from build123d import *

# Parameters (mm, degrees)
SKETCH1_W           = 13.26865531
SKETCH1_H           = 13.268655309
BOSS_EXTRUDE1_DEPTH = 7.62
SKETCH5_R           = 1.27
CUT_EXTRUDE3_DEPTH  = 8.62
CUT_EXTRUDE5_REACH  = 9.62
SKETCH9_W           = 32
SKETCH9_H           = 8.5
SKETCH10_R          = 1.625
CUT_EXTRUDE6_DEPTH  = 8.62
SKETCH13_W          = 21.59
SKETCH13_H          = 6.35
SKETCH13_W_2        = 13.26865531
BOSS_EXTRUDE2_DEPTH = 19.05
SKETCH14_R          = 2.286
CUT_EXTRUDE7_DEPTH  = 201.924200001
SKETCH15_R          = 2.286
CUT_EXTRUDE8_DEPTH  = 123.971427656
SKETCH8_R           = 1.6250031
CUT_EXTRUDE9_DEPTH  = 27.67
SKETCH19_R          = 2.286
CUT_EXTRUDE13_DEPTH = 201.924200001
CUT_EXTRUDE14_REACH = 28.67
SKETCH20_R          = 1.625
SKETCH22_W          = 11.684
SKETCH22_H          = 11.684
SKETCH22_W_2        = 45.3
SKETCH22_H_2        = 36.3
SKETCH22_W_3        = 83.82
SKETCH22_H_3        = 63.500000001
SKETCH22_W_4        = 41.91
SKETCH22_W_5        = 15.24
SKETCH22_H_4        = 100.5942
CUT_EXTRUDE15_DEPTH = 27.67
SKETCH24_R          = 1.625
CUT_EXTRUDE16_DEPTH = 27.67
FILLET2_R           = 6.35
FILLET4_R           = 6.35
FILLET5_R           = 6.35


with BuildPart() as part:
    # Sketch1 → Boss-Extrude1 (new body)
    with BuildSketch(Plane(origin=(0, 0, 0), x_dir=(-1, 0, 0), z_dir=(0, 0, 1))):
        Polygon((0, -67.741156164), (0, -193.735356164), (-21.59, -193.735356164), (-21.59, -215.325356165), (0, -215.325356165), (0, -240.725356165), (-153.67, -240.725356165), (-153.67, -165.028256165), (-195.58, -165.028256165), (-195.58, -89.331156165), (-217.17, -89.331156165), (-217.17, -67.741156164), (-195.58, -67.741156164), (-195.58, -46.151156164), (-217.17, -46.151156164), (-217.17, -20.751156164), (0, -20.751156164), (0, -46.151156164), (-21.59, -46.151156164), (-21.59, -67.741156164), align=None)
        with Locations((-114.925672351, -130.738256165)):
            Rectangle(SKETCH1_W, SKETCH1_H, mode=Mode.SUBTRACT)
    extrude(amount=BOSS_EXTRUDE1_DEPTH)

    # Sketch5 → Cut-Extrude3 (cut, through all)
    with BuildSketch(Plane.XY.offset(7.62)):
        with Locations((44.45, 234.375356165)):
            Circle(SKETCH5_R)
        with Locations((140.97, 234.375356165)):
            Circle(SKETCH5_R)
        with Locations((44.45, 158.175356164)):
            Circle(SKETCH5_R)
        with Locations((140.97, 158.175356164)):
            Circle(SKETCH5_R)
    extrude(amount=-CUT_EXTRUDE3_DEPTH, mode=Mode.SUBTRACT)

    # Sketch9 → Cut-Extrude5 (cut, up to next)
    with BuildSketch(Plane(origin=(0, 0, 0), x_dir=(-1, 0, 0), z_dir=(0, 0, -1)), mode=Mode.PRIVATE) as cut_extrude5_sk1:
        with Locations((-43.94, 33.467738164)):
            Rectangle(SKETCH9_W, SKETCH9_H)
    cut_extrude5_tool1 = extrude(cut_extrude5_sk1.sketch, amount=-CUT_EXTRUDE5_REACH, mode=Mode.PRIVATE) & part.part
    add(cut_extrude5_tool1.solids().sort_by_distance((43.94, 33.467738, 0))[0], mode=Mode.SUBTRACT)

    # Sketch10 → Cut-Extrude6 (cut, through all)
    with BuildSketch(Plane.XY.offset(7.62)):
        with Locations((179.07, 142.930256164)):
            Circle(SKETCH10_R)
        with Locations((179.07, 118.546256164)):
            Circle(SKETCH10_R)
        with Locations((154.686, 118.546256164)):
            Circle(SKETCH10_R)
        with Locations((154.686, 142.930256164)):
            Circle(SKETCH10_R)
    extrude(amount=-CUT_EXTRUDE6_DEPTH, mode=Mode.SUBTRACT)

    # Sketch13 → Boss-Extrude2 (add)
    with BuildSketch(Plane.XY.offset(7.62)):
        with Locations((10.795, 218.500356165)):
            Rectangle(SKETCH13_W, SKETCH13_H)
        with Locations((10.795, 190.560356164)):
            Rectangle(SKETCH13_W, SKETCH13_H)
        with Locations((10.795, 42.976156164)):
            Rectangle(SKETCH13_W, SKETCH13_H)
        with Locations((10.795, 70.916156164)):
            Rectangle(SKETCH13_W, SKETCH13_H)
        with Locations((114.925672351, 140.547583819)):
            Rectangle(SKETCH13_W_2, SKETCH13_H)
        with Locations((114.925672351, 120.92892851)):
            Rectangle(SKETCH13_W_2, SKETCH13_H)
        with Locations((206.375, 42.976156164)):
            Rectangle(SKETCH13_W, SKETCH13_H)
        with Locations((206.375, 70.916156164)):
            Rectangle(SKETCH13_W, SKETCH13_H)
    extrude(amount=BOSS_EXTRUDE2_DEPTH)

    # Sketch14 → Cut-Extrude7 (cut, through all)
    with BuildSketch(Plane.XZ.offset(-39.801156164)):
        with Locations((10.795, 17.145)):
            Circle(SKETCH14_R)
    extrude(amount=-CUT_EXTRUDE7_DEPTH, mode=Mode.SUBTRACT)

    # Sketch15 → Cut-Extrude8 (cut, through all)
    with BuildSketch(Plane.XZ.offset(-117.75392851)):
        with Locations((114.925672351, 17.145)):
            Circle(SKETCH15_R)
    extrude(amount=-CUT_EXTRUDE8_DEPTH, mode=Mode.SUBTRACT)

    # Sketch8 → Cut-Extrude9 (cut, through all)
    with BuildSketch(Plane(origin=(0, 0, 0), x_dir=(-1, 0, 0), z_dir=(0, 0, -1))):
        with Locations((-88.9, 52.501156164)):
            Circle(SKETCH8_R)
        with Locations((-146.9, 52.501156164)):
            Circle(SKETCH8_R)
        with Locations((-88.9, 101.501156164)):
            Circle(SKETCH8_R)
        with Locations((-146.9, 101.501156164)):
            Circle(SKETCH8_R)
    extrude(amount=-CUT_EXTRUDE9_DEPTH, mode=Mode.SUBTRACT)

    # Sketch19 → Cut-Extrude13 (cut, through all)
    with BuildSketch(Plane.XZ.offset(-39.801156164)):
        with Locations((206.375, 17.145)):
            Circle(SKETCH19_R)
    extrude(amount=-CUT_EXTRUDE13_DEPTH, mode=Mode.SUBTRACT)

    # Sketch20 → Cut-Extrude14 (cut, up to next)
    with BuildSketch(Plane(origin=(0, 0, 0), x_dir=(-1, 0, 0), z_dir=(0, 0, -1)), mode=Mode.PRIVATE) as cut_extrude14_sk1:
        with Locations((-81.741344696, 139.338256164)):
            Circle(SKETCH20_R)
    cut_extrude14_tool1 = extrude(cut_extrude14_sk1.sketch, amount=-CUT_EXTRUDE14_REACH, mode=Mode.PRIVATE) & part.part
    add(cut_extrude14_tool1.solids().sort_by_distance((81.741345, 139.338256, 0))[0], mode=Mode.SUBTRACT)
    # Sketch20 → Cut-Extrude14 (cut, up to next)
    with BuildSketch(Plane(origin=(0, 0, 0), x_dir=(-1, 0, 0), z_dir=(0, 0, -1)), mode=Mode.PRIVATE) as cut_extrude14_sk2:
        with Locations((-54.241344696, 122.138256164)):
            Circle(SKETCH20_R)
    cut_extrude14_tool2 = extrude(cut_extrude14_sk2.sketch, amount=-CUT_EXTRUDE14_REACH, mode=Mode.PRIVATE) & part.part
    add(cut_extrude14_tool2.solids().sort_by_distance((54.241345, 122.138256, 0))[0], mode=Mode.SUBTRACT)

    # Sketch22 → Cut-Extrude15 (cut, through all)
    with BuildSketch(Plane(origin=(0, 0, 0), x_dir=(-1, 0, 0), z_dir=(0, 0, -1))):
        with Locations((-166.878, 130.738256164)):
            Rectangle(SKETCH22_W, SKETCH22_H)
        with Locations((-117.9, 77.001156164)):
            Rectangle(SKETCH22_W_2, SKETCH22_H_2)
        with Locations((-92.71, 196.275356165)):
            Rectangle(SKETCH22_W_3, SKETCH22_H_3)
        with Locations((-61.595, 77.001156164)):
            Rectangle(SKETCH22_W_4, SKETCH22_H_2)
        with Locations((-20.32, 130.738256164)):
            Rectangle(SKETCH22_W_5, SKETCH22_H_4)
    extrude(amount=-CUT_EXTRUDE15_DEPTH, mode=Mode.SUBTRACT)

    # Sketch24 → Cut-Extrude16 (cut, through all)
    with BuildSketch(Plane(origin=(0, 0, 0), x_dir=(-1, 0, 0), z_dir=(0, 0, -1))):
        with Locations((-179.07, 101.501156164)):
            Circle(SKETCH24_R)
        with Locations((-159.07, 101.501156164)):
            Circle(SKETCH24_R)
        with Locations((-159.07, 52.501156164)):
            Circle(SKETCH24_R)
        with Locations((-179.07, 52.501156164)):
            Circle(SKETCH24_R)
    extrude(amount=-CUT_EXTRUDE16_DEPTH, mode=Mode.SUBTRACT)

    # Fillet2
    fillet2_edges = [part.edges().sort_by_distance(p)[0] for p in [
        (0, 218.500356165, 26.67),
        (21.59, 218.500356165, 26.67),
        (0, 190.560356164, 26.67),
        (21.59, 190.560356164, 26.67),
        (0, 42.976156164, 26.67),
        (21.59, 42.976156164, 26.67),
        (0, 70.916156164, 26.67),
        (21.59, 70.916156164, 26.67),
        (121.560000006, 120.92892851, 26.67),
        (108.291344696, 120.92892851, 26.67),
        (121.560000006, 140.547583819, 26.67),
        (108.291344696, 140.547583819, 26.67),
        (217.17, 70.916156164, 26.67),
        (195.58, 70.916156164, 26.67),
        (217.17, 42.976156164, 26.67),
        (195.58, 42.976156164, 26.67),
    ]]
    fillet(fillet2_edges, radius=FILLET2_R)

    # Fillet4
    fillet4_edges = [part.edges().sort_by_distance(p)[0] for p in [
        (0, 20.751156164, 3.81),
        (217.17, 20.751156164, 3.81),
        (217.17, 89.331156165, 3.81),
        (195.58, 89.331156165, 3.81),
        (195.58, 165.028256165, 3.81),
        (153.67, 165.028256165, 3.81),
        (153.67, 240.725356165, 3.81),
        (0, 240.725356165, 3.81),
    ]]
    fillet(fillet4_edges, radius=FILLET4_R)

    # Fillet5
    fillet5_edges = [part.edges().sort_by_distance(p)[0] for p in [
        (27.94, 80.441156164, 3.81),
        (27.94, 181.035356164, 3.81),
        (12.7, 181.035356164, 3.81),
        (12.7, 80.441156164, 3.81),
        (82.55, 58.851156164, 3.81),
        (82.55, 95.151156164, 3.81),
        (40.64, 95.151156164, 3.81),
        (40.64, 58.851156164, 3.81),
        (134.62, 164.525356164, 3.81),
        (134.62, 228.025356165, 3.81),
        (50.8, 228.025356165, 3.81),
        (50.8, 164.525356164, 3.81),
        (140.55, 58.851156164, 3.81),
        (140.55, 95.151156164, 3.81),
        (95.25, 95.151156164, 3.81),
        (95.25, 58.851156164, 3.81),
    ]]
    fillet(fillet5_edges, radius=FILLET5_R)


solid = part.part
Work out the finished part from the listing and answer in its coordinate system (mm). A direction names the side the tool comes from. Give positions to 0.01 mm unless a question says otherwise; leave off trailing zeros. Order: outer loops, then holes, each group sorted by start corner. A loop starts at its lowest first (then second) coordinate and runs counter-clockwise, first axis right, second up. Notation, with made-up numbers: (67.5, -35.75) -> (92.5, -35.75) arc R19 cw to (92.5, -17.75) -> close; hole circle Ø6 at (87, 46). An arc over 180 degrees is marked (long way). Answer as a JSON object with one key per item and string values. Group by question number.
1. Section A-A on z = 10.5 is taken. Count the separate pieces of the cut face and the enclosed holes in it, plus the area to 3 significant figures.
2. A tool of negligible diameter and unlimited length cuts with its end or side. For faces 1 (the flat face through (27.94, 130, 4)), 2 (the flat face through (11, 215.325, 13)), 3 (the flat face through (207, 67.741, 13)), 4 (the flat face through (108.291, 141, 14)), from which of +Z, -Z, +X, -X, +Y, -Y can it reach the whole face along a straight path? Write none if from no direction.
3. Section B-B on y = 34.5 is taken. Determine the outline of the cut face in (x, z), plus the area to 3 significant figures.
4. Section C-C on x = 168 is taken. Determine the outline of the cut face in (y, z).
5. Flat-ended cylindrical pins translate along their axes: pin 1 Ø8.5 at (y, z) = (202.5, 4) entering from -X; pin 2 Ø11 at (x, z) = (211.5, 15) entering from -Y; pin 3 Ø3 at (x, y) = (142, 172) entering from +Z; pin 4 Ø5 at (x, z) = (193, 14.5) entering from -Y. Find the tip coordinate at first contact, or state that the pin passes through.
6. Consider line 1 along Y through (x, z) = (111, 2); line 2 along Y through (x, z) = (79, 3); line 3 along X through (y, z) = (45.5, 16.25). Determine where each line is inside the solid, lowest interval first. Write a range as [from, to].
7. The mould has two halves that part along X. Classify faces 5 (the cylindrical face through (138.74, 93.24, 3.86)), 6 (the cylindrical face through (1.81, 218.54, 24.76)), 7 (the flat face through (8, 187.385, 17)): released by +X, released by -X, zero draft, split by the parting line, or undercut.
Result sheet:
{
 "1": {"separate pieces": "8", "enclosed holes": "0", "area": "991 mm^2"},
 "2": {"face 1": "+Z, -Z", "face 2": "+Z, -Z, -X", "face 3": "+Z, -Z, +X", "face 4": "+Z, -X, +Y, -Y"},
 "3": {"outline": "(0, 0) -> (27.94, 0) -> (27.94, 7.62) -> (0, 7.62) -> close; (59.94, 0) -> (217.17, 0) -> (217.17, 7.62) -> (59.94, 7.62) -> close", "area": "1,410 mm^2"},
 "4": {"outline": "(20.75, 0) -> (124.9, 0) -> (124.9, 7.62) -> (20.75, 7.62) -> close; (136.58, 0) -> (165.03, 0) -> (165.03, 7.62) -> (136.58, 7.62) -> close"},
 "5": {"pin 1": "stops at x = 21.59", "pin 2": "stops at y = 39.8", "pin 3": "stops at z = 7.62", "pin 4": "passes through"},
 "6": {"line 1": "y = [20.75, 58.85], [95.15, 124.1], [137.37, 164.53], [228.03, 240.73]", "line 2": "y = [20.75, 59.5], [94.5, 164.53], [228.03, 240.73]", "line 3": "x = [0, 8.69], [12.9, 21.59], [195.58, 204.27], [208.48, 217.17]"},
 "7": {"face 5": "undercut", "face 6": "released by -X", "face 7": "zero draft"}
}
